from build123d import *

# Parameters (mm, degrees)
ESQUISSE2_W                             = 360
ESQUISSE2_H                             = 30
T_LE_DE_BASE_PLI_E1_DEPTH               = 3
T_LE_PLI_E_SUR_AR_TE1_STRIP_W           = 18
T_LE_PLI_E_SUR_AR_TE1_STRIP_H           = 3
T_LE_PLI_E_SUR_AR_TE1_STRIP_CUT_DEPTH   = 360
T_LE_PLI_E_SUR_AR_TE1_STRIP_2_W         = 18
T_LE_PLI_E_SUR_AR_TE1_STRIP_2_H         = 3
T_LE_PLI_E_SUR_AR_TE1_STRIP_CUT_2_DEPTH = 360
T_LE_PLI_E_SUR_AR_TE1_DEPTH             = 360
T_LE_PLI_E_SUR_AR_TE1_BEND_DEPTH        = 360
ENL_V_MAT_EXTRU_1_REACH                 = 363.447
ESQUISSE10_R                            = 4


# Sheet-metal steps are written as plain solids
with BuildPart() as part:
    # Esquisse2 → Tôle de base pliée1 (new body)
    with BuildSketch(Plane(origin=(0, 0, 0), x_dir=(1, 0, 0), z_dir=(0, 1, 0))):
        with Locations((180, 15)):
            Rectangle(ESQUISSE2_W, ESQUISSE2_H)
    extrude(amount=-T_LE_DE_BASE_PLI_E1_DEPTH)

    # Tôle pliée sur arête1 strip (across the edge) → Tôle pliée sur arête1 strip cut (cut)
    with BuildSketch(Plane(origin=(0, 0, 0), x_dir=(0, 0, -1), z_dir=(1, 0, 0))):
        with Locations((-3, -1.5)):
            Rectangle(T_LE_PLI_E_SUR_AR_TE1_STRIP_W, T_LE_PLI_E_SUR_AR_TE1_STRIP_H)
    extrude(amount=T_LE_PLI_E_SUR_AR_TE1_STRIP_CUT_DEPTH, mode=Mode.SUBTRACT)

    # Tôle pliée sur arête1 strip 2 (across the edge) → Tôle pliée sur arête1 strip cut 2 (cut)
    with BuildSketch(Plane(origin=(360, 0, -30), x_dir=(0, 0, 1), z_dir=(-1, 0, 0))):
        with Locations((-3, -1.5)):
            Rectangle(T_LE_PLI_E_SUR_AR_TE1_STRIP_2_W, T_LE_PLI_E_SUR_AR_TE1_STRIP_2_H)
    extrude(amount=T_LE_PLI_E_SUR_AR_TE1_STRIP_CUT_2_DEPTH, mode=Mode.SUBTRACT)

    # Tôle pliée sur arête1 section (across the edge) → Tôle pliée sur arête1 (add)
    with BuildSketch(Plane(origin=(0, 0, 0), x_dir=(0, 0, -1), z_dir=(1, 0, 0))):
        with BuildLine():
            Line((0, 3), (0, 12))
            Line((0, 12), (3, 12))
            Line((3, 12), (3, 3))
            ThreePointArc((3, 3), (3.878679656, 0.878679656), (6, 0))
            Line((6, 0), (6, -3))
            ThreePointArc((6, -3), (1.757359313, -1.242640687), (0, 3))
        make_face()
    extrude(amount=T_LE_PLI_E_SUR_AR_TE1_DEPTH)

    # Tôle pliée sur arête1 section 2 (across the edge) → Tôle pliée sur arête1 bend (add)
    with BuildSketch(Plane(origin=(360, 0, -30), x_dir=(0, 0, 1), z_dir=(-1, 0, 0))):
        with BuildLine():
            Line((0, 3), (0, 12))
            Line((0, 12), (3, 12))
            Line((3, 12), (3, 3))
            ThreePointArc((3, 3), (3.878679656, 0.878679656), (6, 0))
            Line((6, 0), (6, -3))
            ThreePointArc((6, -3), (1.757359313, -1.242640687), (0, 3))
        make_face()
    extrude(amount=T_LE_PLI_E_SUR_AR_TE1_BEND_DEPTH)

    # Esquisse10 → Enlèv. mat.-Extru.1 (cut, up to next)
    with BuildSketch(Plane(origin=(0, 0, 0), x_dir=(1, 0, 0), z_dir=(0, 1, 0)), mode=Mode.PRIVATE) as enl_v_mat_extru_1_sk1:
        with Locations(Location((15, 15, 0), (0, 0, 270))):
            Circle(ESQUISSE10_R)
    enl_v_mat_extru_1_tool1 = extrude(enl_v_mat_extru_1_sk1.sketch, amount=-ENL_V_MAT_EXTRU_1_REACH, mode=Mode.PRIVATE) & part.part
    # Esquisse10 → Enlèv. mat.-Extru.1 (cut, up to next)
    with BuildSketch(Plane(origin=(0, 0, 0), x_dir=(1, 0, 0), z_dir=(0, 1, 0)), mode=Mode.PRIVATE) as enl_v_mat_extru_1_sk2:
        with Locations(Location((345, 15, 0), (0, 0, 270))):
            Circle(ESQUISSE10_R)
    enl_v_mat_extru_1_tool2 = extrude(enl_v_mat_extru_1_sk2.sketch, amount=-ENL_V_MAT_EXTRU_1_REACH, mode=Mode.PRIVATE) & part.part
    add(enl_v_mat_extru_1_tool1.solids().sort_by_distance((15, 0, -15))[0], mode=Mode.SUBTRACT)
    add(enl_v_mat_extru_1_tool2.solids().sort_by_distance((345, 0, -15))[0], mode=Mode.SUBTRACT)


solid = part.part
Work out the finished part from the listing and answer in its coordinate system (mm). A direction names the side the tool comes from. Give positions to 0.01 mm unless a question says otherwise; leave off trailing zeros. Order: outer loops, then holes, each group sorted by start corner. A loop starts at its lowest first (then second) coordinate and runs counter-clockwise, first axis right, second up. Notation, with made-up numbers: (19, 76) -> (28, 76) arc R4 ccw to (28, 82) -> close; hole circle Ø7 at (10.5, -21.5). An arc over 180 degrees is marked (long way). Answer as a JSON object with one key per item and string values. Group by question number.
1. Section C-C on x = 109.5 is taken. Determine the outline of the cut face in (y, z).
2. Section A-A on x = 15 is taken. Determine the outline of the cut face in (y, z), plus the area to 3 significant figures.
3. Section B-B on z = -15 is taken. Determine the outline of the cut face in (x, y).
4. Flat-ended cylindrical pins translate along their axes: pin 1 Ø5.5 at (x, z) = (261.5, -10.5) entering from +Y; pin 2 Ø6 at (y, z) = (2.5, -12) entering from +X. Find the tip coordinate at first contact, or state that the pin passes through.
5. Consider line 1 along X through (y, z) = (-1.25, -15); line 2 along Z through (x, y) = (335, 5.5); line 3 along Y through (x, z) = (84, -15.5). Determine where each line is inside the solid, lowest interval first. Write a range as [from, to].
6. A tool of negligible diameter and unlimited length cuts with its end or side. For faces 1 (the flat face through (183, 7, -30)), 2 (the flat face through (177, 8, -3)), from which of +Z, -Z, +X, -X, +Y, -Y can it reach the whole face along a straight path? Write none if from no direction.
7. The mould has two halves that part along X. Classify faces 3 (the flat face through (360, -0.4, -14.8)), 4 (the flat face through (183, 8, -27)), 5 (the cylindrical face through (17.7, -1.48, -17.95)), 6 (the flat face through (0, -0.4, -14.8)): released by +X, released by -X, zero draft, split by the parting line, or undercut.
Result sheet:
{
 "1": {"outline": "(-3, -24) arc R6 ccw to (3, -30) -> (12, -30) -> (12, -27) -> (3, -27) arc R3 cw to (0, -24) -> (0, -6) arc R3 cw to (3, -3) -> (12, -3) -> (12, 0) -> (3, 0) arc R6 ccw to (-3, -6) -> close"},
 "2": {"outline": "(-3, -24) arc R6 ccw to (3, -30) -> (12, -30) -> (12, -27) -> (3, -27) arc R3 cw to (0, -24) -> (0, -19) -> (-3, -19) -> close; (-3, -11) -> (0, -11) -> (0, -6) arc R3 cw to (3, -3) -> (12, -3) -> (12, 0) -> (3, 0) arc R6 ccw to (-3, -6) -> close", "area": "126 mm^2"},
 "3": {"outline": "(0, -3) -> (11, -3) -> (11, 0) -> (0, 0) -> close; (19, -3) -> (341, -3) -> (341, 0) -> (19, 0) -> close; (349, -3) -> (360, -3) -> (360, 0) -> (349, 0) -> close"},
 "4": {"pin 1": "stops at y = 0", "pin 2": "stops at x = 360"},
 "5": {"line 1": "x = [0, 11], [19, 341], [349, 360]", "line 2": "z = [-30, -27], [-3, 0]", "line 3": "y = [-3, 0]"},
 "6": {"face 1": "-Z, +X, -X, +Y, -Y", "face 2": "+X, -X, +Y"},
 "7": {"face 3": "released by +X", "face 4": "zero draft", "face 5": "undercut", "face 6": "released by -X"}
}
